from build123d import *

# Parameters (mm, degrees)
F1_DEPTH = 36
F2_R     = 8
F3_DEPTH = 32
F4_R     = 8
F5_DEPTH = 29.001
F6_R     = 8
F7_DEPTH = 29.001
F8_D     = 16
F9_R     = 16


with BuildPart() as f1:
    # F0 (on Front) → F1 (new body)
    with BuildSketch(Plane.XZ):
        Polygon((19.2118563248, 11), (-33.2294469934, 11), (-33.2294469934, 0), (8.2118563248, 0), (8.2118563248, -18), (-33.2294469934, -18), (-33.2294469934, -29), (19.2118563248, -29), (19.2118563248, -18), (19.2118563248, 0), align=None)
    extrude(amount=F1_DEPTH)

    # F2 (on face) → F3 (join)
    with BuildSketch(Plane.YZ.offset(19.2118563248)):
        with Locations((-18, -9)):
            Circle(F2_R)
    extrude(amount=F3_DEPTH)

    # F4 (on Top) → F5 (cut, through all)
    with BuildSketch(Plane.XY):
        with Locations((-16.9795084218, -18.1846376508)):
            Circle(F4_R)
    extrude(amount=-F5_DEPTH, mode=Mode.SUBTRACT)

    # F6 (on Top) → F7 (cut, through all)
    with BuildSketch(Plane.XY):
        with Locations((-17.4762796468, -18.1846376508)):
            Circle(F6_R)
    extrude(amount=-F7_DEPTH, mode=Mode.SUBTRACT)

    # F8 (through all)
    with Locations(Plane(origin=(0, 0, 0), x_dir=(1, 0, 0), z_dir=(0, 0, -1))):
        with Locations((-16.9795084218, 18.1846376508)):
            Hole(F8_D / 2)

    # F9
    f9_edges = [f1.edges().sort_by_distance(p)[0] for p in [
        (-33.229447, 0, -23.5),
        (-33.229447, 0, 5.5),
        (-33.229447, -36, 5.5),
        (-33.229447, -36, -23.5),
    ]]
    fillet(f9_edges, radius=F9_R)


solid = f1.part
The listing builds one solid part. Answer for the finished solid, in the listing's coordinates (mm). A direction names the side the tool comes from. Give positions to 0.01 mm unless a question says otherwise; leave off trailing zeros. Write each loop counter-clockwise with the first axis right and the second up, starting at its lowest first coordinate (ties: lowest second). Pieces come first, ordered by that corner, then holes.
Item 1: Find the intervals of material crossed by line 1 along Z through (x, y) = (-19, -6.5); line 2 along X through (y, z) = (-18, -22); line 3 along X through (y, z) = (-18, -0.5), in increasing order.
Item 2: Determine the mould class of faces 1 (the cylindrical face through (-25.474, -18.005, -23.423)), 2 (the flat face through (8.212, -18, -9)), 3 (the flat face through (-8, -18, 0)) for opening direction X: released by +X, released by -X, zero draft, split by the parting line, or undercut.
Item 3: Section A-A, the plane y = -13 is taken. Write down the section's boundary in (x, z) (3 decimals).
Item 4: Section B-B, the plane z = -9 is taken. Write down the section's boundary in (x, y).
Item 5: Section D-D, the plane y = -31.5 is taken. Write down the section's boundary in (x, z), plus the area to 3 significant figures.
Item 6: Section C-C, the plane x = -20.5 is taken. Write down the section's boundary in (y, z), plus the area to 3 significant figures.
Item 7: Which of the six approach directions +Z, -Z, +X, -X, +Y, -Y give full straight-line access (tool end or side, diameter ignored) to faces 4 (the flat face through (-8, -18, -18)), 5 (the cylindrical face through (35, -26, -9)), 6 (the cylindrical face through (-8.98, -18.36, -23.42))?
Item 8: Flat-ended cylindrical pins translate along their axes: P1, Ø12, axis at y = -21.5, z = -1, coming from the +X side; P2, Ø5.5, axis at y = -24.5, z = -13, coming from the -X side; P3, Ø8, axis at y = -16, z = 6, coming from the +X side. Find the tip coordinate at first contact, or state that the pin passes through.
Completed:
1. line 1: z = -29 to -18, 0 to 11
1. line 2: x = -33.23 to -25.47, -8.98 to 19.21
1. line 3: x = 8.21 to 19.21
2. face 1: undercut
2. face 2: released by -X
2. face 3: zero draft
3. outline: (-32.946, -29) - (-23.569, -29) - (-23.569, -18) - (-32.946, -18) - close; (-32.946, 0) - (-23.072, 0) - (-23.072, 11) - (-32.946, 11) - close; (-10.887, -29) - (19.212, -29) - (19.212, -15.245) - (51.212, -15.245) - (51.212, -2.755) - (19.212, -2.755) - (19.212, 11) - (-10.887, 11) - (-10.887, 0) - (8.212, 0) - (8.212, -18) - (-10.887, -18) - close
4. outline: (8.21, -36) - (19.21, -36) - (19.21, -26) - (51.21, -26) - (51.21, -10) - (19.21, -10) - (19.21, 0) - (8.21, 0) - close
5. outline: (-28.35, -29) - (19.21, -29) - (19.21, 11) - (-28.35, 11) - (-28.35, 0) - (8.21, 0) - (8.21, -18) - (-28.35, -18) - close
5. area: 1,240 mm2
6. outline: (-35.66, -29) - (-25.59, -29) - (-25.59, -18) - (-35.66, -18) - close; (-35.66, 0) - (-25.37, 0) - (-25.37, 11) - (-35.66, 11) - close; (-11, 0) - (-0.34, 0) - (-0.34, 11) - (-11, 11) - close; (-10.78, -29) - (-0.34, -29) - (-0.34, -18) - (-10.78, -18) - close
6. area: 456 mm2
7. face 4: -X, +Y, -Y
7. face 5: +X
7. face 6: +Z, -Z
8. P1: stops at x = 51.21
8. P2: stops at x = 8.21
8. P3: stops at x = 19.21
